Print and shaded views of the part. All mm, measured from the part's lowest x, y and z. A direction names the side the tool comes from. Round coordinates to 2 decimals unless told otherwise and drop trailing zeros. Loops run counter-clockwise (first coordinate to the right, second up) from the corner with the lowest first, then second, coordinate; pieces in that order, holes last. Notation, with made-up numbers: (36, 57.5) - (67, 57.5) arc R12 ccw to (67, 61.5) - close; hole circle Ø4 at (28.25, 12). An arc over 180 degrees is marked (long way). Use one line per item in the form item = value.
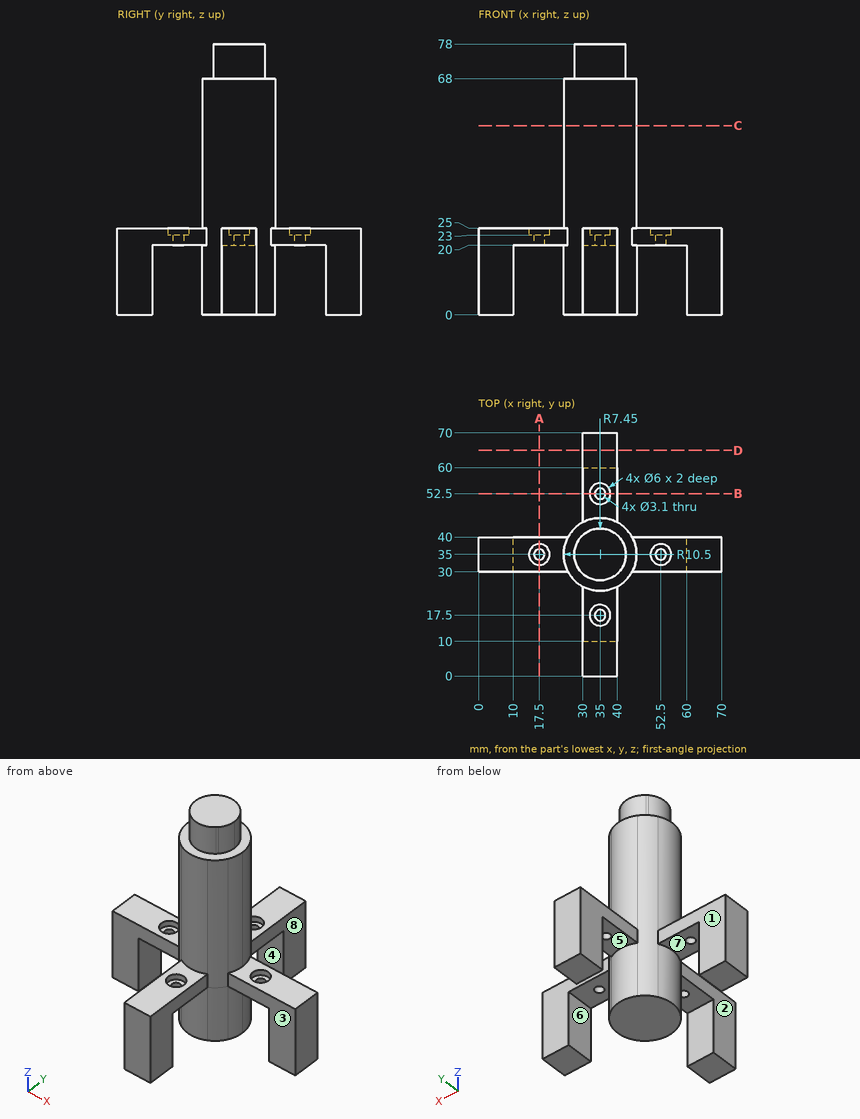
1. Pull direction X, two halves, no side cores. Call the marked faces 5, 6, 7 and 8: +X half, -X half, draft (parallel to the pull), parting line (faces both ways), or undercut.
Geometry check:
face_5 = draft
face_6 = undercut
face_7 = undercut
face_8 = +X half
2. Tool access for the marked faces 1, 2, 3 and 4: list every direction of +Z, -Z, +X, -X, +Y, -Y with a clear straight run to the whole face (end or side of a thin tool).
Geometry check:
face_1 = +Z, -Z, -X, +Y
face_2 = +Z, -Z, -X, -Y
face_3 = +Z, -Z, +X, -Y
face_4 = -Z, +X, -X
3. Flat gauge pins, fed straight in: pin 1 (5 mm diameter, centred on x = 19.5, y = 36, fed in from -Z); pin 2 (2 mm diameter, centred on y = 24, z = 24, fed in from +X); pin 3 (11 mm diameter, centred on x = 36, z = 13.5, fed in from -Y); pin 4 (6.5 mm diameter, centred on x = 34, y = 53.5, fed in from +Z). Where does each tip first touch, or does it go through?
Geometry check:
pin_1 = 20
pin_2 = 40
pin_3 = 0
pin_4 = 25
4. Wall check: probe 1 along Y at (x, z) = (35, 22.2); probe 2 along X at (y, z) = (35, 4.5); probe 3 along Y at (x, z) = (17.5, 23.95). Give the ranges that are in metal, low to high.
Geometry check:
probe_1 = 0 to 15.95, 19.05 to 50.95, 54.05 to 70
probe_2 = 0 to 10, 24.5 to 45.5, 60 to 70
probe_3 = 30 to 32, 38 to 40
5. Cut at D-D, the plane y = 65. Give the cut face in (x, z).
Geometry check:
outline = (30, 0) - (40, 0) - (40, 25) - (30, 25) - close
6. Cut at C-C, the plane z = 54.5. Give the cut face in (x, y), plus the area to 3 significant figures.
Geometry check:
outline = circle Ø21 at (35, 35)
area = 346 mm^2
7. Cut at A-A, the plane x = 17.5. Give the cut face in (y, z).
Geometry check:
outline = (30, 20) - (33.45, 20) - (33.45, 23) - (32, 23) - (32, 25) - (30, 25) - close; (36.55, 20) - (40, 20) - (40, 25) - (38, 25) - (38, 23) - (36.55, 23) - close
